Can you work these out from the model? Positions are in its coordinate system, mm. Coordinates: 2 decimals unless noted, no trailing zeros. Answer as a JSON object with one key per item and string values.
from build123d import *

# Parameters (mm, degrees)
SKETCH1_W           = 80.518
SKETCH1_H           = 80.518
BOSS_EXTRUDE1_DEPTH = 24.9936
SKETCH2_R           = 2.032
CUT_EXTRUDE1_DEPTH  = 117.580344351


with BuildPart() as part:
    # Sketch1 → Boss-Extrude1 (new body)
    with BuildSketch(Plane(origin=(0, 0, 0), x_dir=(1, 0, 0), z_dir=(0, 1, 0))):
        with Locations((40.259, 40.259)):
            Rectangle(SKETCH1_W, SKETCH1_H)
    extrude(amount=BOSS_EXTRUDE1_DEPTH)

    # Sketch2 → Cut-Extrude1 (cut, through all)
    with BuildSketch(Plane(origin=(0, 24.9936, 0), x_dir=(1, 0, 0), z_dir=(0, 1, 0))):
        with Locations(Location((4.572, 75.946, 0), (0, 0, 270))):
            Circle(SKETCH2_R)
        with Locations(Location((75.946, 75.946, 0), (0, 0, 270))):
            Circle(SKETCH2_R)
    cut_extrude1 = extrude(amount=-CUT_EXTRUDE1_DEPTH, mode=Mode.SUBTRACT)

    # Mirror1: Cut-Extrude1 across plane
    add(cut_extrude1.mirror(Plane(origin=(0, 0, -40.259), x_dir=(1, 0, 0), z_dir=(0, 0, -1))), mode=Mode.SUBTRACT)


solid = part.part
Item 1: Please list where this line runs through material, in increasing order: line 1 (X direction, y = 23.5, z = -6).
Answers follow:
{"line 1": "x = 0 to 3.13, 6.02 to 74.5, 77.39 to 80.52"}
Item 2: I'm going to push flat-ended pins straight in: pin 1 (2.5 mm diameter, centred on x = 75.946, z = -75.946, fed in from -Y); pin 2 (4 mm diameter, centred on x = 49.5, y = 19.5, fed in from +Z). Where does each tip first touch, or does it pass through?
Answers follow:
{"pin 1": "passes through", "pin 2": "stops at z = 0"}
Item 3: If we mould it in two halves opening along Z, with no side actions, what happens to faces 1 (the cylindrical face through (75.17, 12.67, -74.07)), 2 (the flat face through (0, 12, -40)), 3 (the flat face through (40, 12, 0))? For each: pulls with the +Z half, pulls with the -Z half, needs draft (parallel to the pull), parting line crosses it, or undercut.
Answers follow:
{"face 1": "undercut", "face 2": "needs draft", "face 3": "pulls with the +Z half"}
